Autodesk Inventor part; units mm, degrees
ref_plane "YZ Plane" through (0, 0, 0) normal (1, 0, 0) x (0, 1, 0)
ref_plane "XZ Plane" through (0, 0, 0) normal (0, 1, 0) x (-1, 0, 0)
ref_plane "XY Plane" through (0, 0, 0) normal (0, 0, 1) x (1, 0, 0)
sketch "Sketch1" plane through (0, 0, 0) normal (0, 0, 1) x (1, 0, 0)
  point P0 (0, 0)
sketch "Sketch2" plane through (0, 0, 0) normal (0, 0, 1) x (1, 0, 0)
  circle A0 centre (0, 0) radius 3.4
  dimension "d0" = 6.8
extrude "Extrusion1" add sketch "Sketch2" along normal blind 4
sketch "Sketch3" plane through (0, 0, 4) normal (0, 0, 1) x (1, 0, 0)
  circle A0 centre (0, 0) radius 3.4
  circle A1 centre (0, 0) radius 1.9
  dimension "d3" = 3.8
extrude "Extrusion2" add sketch "Sketch3" along normal blind 15.7 contours A1
sketch "Sketch4" plane through (0, 0, 0) normal (0, 0, -1) x (-1, 0, 0)
  circle A0 centre (0, 0) radius 3.4
  circle A1 centre (0, 0) radius 3.4
  line L0 (-0.8625, 1.4939) -> (0.8625, 1.4939)
  line L1 (0.8625, 1.4939) -> (1.725, 0)
  line L2 (1.725, 0) -> (0.8625, -1.4939)
  line L3 (0.8625, -1.4939) -> (-0.8625, -1.4939)
  line L4 (-1.725, 0) -> (-0.8625, -1.4939)
  line L5 (-1.725, 0) -> (-0.8625, 1.4939)
extrude "Extrusion3" cut sketch "Sketch4" against normal blind 2.45 contours L0 L1 L2 L3 L4 L5
fillet "Fillet1" radius 0.2 6 edges at (1.2937, 0.7469, 0) (0, 1.4939, 0) (-1.2937, 0.7469, 0) (-1.2937, -0.7469, 0) (0, -1.4939, 0) (1.2937, -0.7469, 0)
fillet "Fillet2" radius 0.2 2 edges at (-3.4, 0, 0) (-3.4, 0, 4)
chamfer "Chamfer1" distance 0.5 angle 45 1 edges at (-1.9, 0, 19.7)
properties part number "LUC GIAC"
Source: CAD feature listing. Evaluate the final solid. Frame: model axes, mm. A direction names the side the tool comes from. Give positions to 0.01 mm unless a question says otherwise; leave off trailing zeros. Loops run counter-clockwise (first coordinate to the right, second up) from the corner with the lowest first, then second, coordinate; pieces in that order, holes last. Notation, with made-up numbers: (-39, 7.25) -> (-12, 7.25) arc R19 ccw to (-12, 17.25) -> close; hole circle Ø11 at (87, 73). An arc over 180 degrees is marked (long way). Use a Markdown table: item, result. Add a question column.
(1) Section query A-A (x = 0). Output: boundary loops of the cut face in (y, z), then the cut area to 3 significant figures.
(2) Access query for faces 4 (the face through (-1.288, 0.757, 1.309)), 5 (the face through (-1.9, -0.08, 11.49)), 6 (the face through (1.4, -1.4, 0)). Directions: +Z, -Z, +X, -X, +Y, -Y. A direction counts if a zero-diameter tool reaches every point of the face in a straight line with its end or side. Return the directions, or none.
(3) Pull-direction query (Y, two-part tool) for faces 1 (the face through (-0.74, 3.32, 1.97)), 2 (the face through (-1.353, 0.765, 0.057)), 3 (the face through (0, 0, 19.7)); classes: +Y half, -Y half, draft (parallel to the pull), parting line (faces both ways), or undercut.
(4) Ray query, line 1 (Z direction, x = 2, y = -2.5); line 2 (Z direction, x = -0.25, y = -1); line 3 (Y direction, x = 1.25, z = 2). Return the intervals inside material, ascending.
(5) Section query C-C (z = 13.5). Output: boundary loops of the cut face in (x, y).
(6) Section query B-B (z = 2.75). Output: boundary loops of the cut face in (x, y).
(7) First-contact query: pin 1 Ø2 at (y, z) = (2.5, 8.5) entering from +X; pin 2 Ø1 at (x, y) = (-0.5, 2) entering from +Z; pin 3 Ø2 at (y, z) = (-1, 9.5) entering from -X; pin 4 Ø4 at (x, y) = (0.5, 2.5) entering from -Z. Flat tips, straight axial feed; report the tip coordinate or a pass-through.
Checked values:
| question | item | result |
|---|---|---|
| 1 | outline | (-3.4, 0.2) arc R0.2 ccw to (-3.2, 0) -> (-1.69, 0) arc R0.2 ccw to (-1.49, 0.2) -> (-1.49, 2.45) -> (1.49, 2.45) -> (1.49, 0.2) arc R0.2 ccw to (1.69, 0) -> (3.2, 0) arc R0.2 ccw to (3.4, 0.2) -> (3.4, 3.8) arc R0.2 ccw to (3.2, 4) -> (1.9, 4) -> (1.9, 19.2) -> (1.4, 19.7) -> (-1.4, 19.7) -> (-1.9, 19.2) -> (-1.9, 4) -> (-3.2, 4) arc R0.2 ccw to (-3.4, 3.8) -> close |
| 1 | area | 79.2 mm^2 |
| 2 | face 4 | -Z |
| 2 | face 5 | +Z |
| 2 | face 6 | -Z, +X, -X, +Y, -Y |
| 3 | face 1 | parting line |
| 3 | face 2 | undercut |
| 3 | face 3 | draft |
| 4 | line 1 | 0 to 4 |
| 4 | line 2 | 2.45 to 19.7 |
| 4 | line 3 | -3.16 to -0.82, 0.82 to 3.16 |
| 5 | outline | circle Ø3.8 at (0, 0) |
| 6 | outline | circle Ø6.8 at (0, 0) |
| 7 | pin 1 | x = 1.17 |
| 7 | pin 2 | z = 19.54 |
| 7 | pin 3 | x = -1.9 |
| 7 | pin 4 | z = 0 |
